from build123d import *

# Parameters (mm, degrees)
F1_DEPTH = 82.55
F2_T     = -3.175
F5_DEPTH = 3.175
F6_DEPTH = 3.175


with BuildPart() as f1:
    # F0 (on Top) → F1 (new body)
    with BuildSketch(Plane.XY):
        Polygon((-132.221535, 93.801795), (-132.221535, 90.626795), (-132.221535, -188.773205), (-132.221535, -191.948205), (115.428465, -191.948205), (115.428465, -188.773205), (115.428465, 93.801795), (112.253465, 93.801795), align=None)
    extrude(amount=F1_DEPTH)

    # F2
    f2_openings = [f1.faces().sort_by_distance(p)[0] for p in [
        (-8.396535, -49.073205, 82.55),
    ]]
    offset(amount=F2_T, openings=f2_openings)

    # F3 (on face) → F5 (join)
    with BuildSketch(Plane.YZ.offset(115.428465)):
        with BuildLine():
            ThreePointArc((52.526795, 53.975), (43.546539, 32.294744), (65.226795, 41.275))
            ThreePointArc((65.226795, 41.275), (61.507051, 50.255256), (52.526795, 53.975))
        make_face()
    extrude(amount=F5_DEPTH)

    # F4 (on face) → F6 (join)
    with BuildSketch(Plane(origin=(-132.221535, 0, 0), x_dir=(0, -1, 0), z_dir=(-1, 0, 0))):
        with BuildLine():
            ThreePointArc((-52.526795, 53.975), (-61.507051, 50.255256), (-65.226795, 41.275))
            ThreePointArc((-65.226795, 41.275), (-52.526795, 28.575), (-39.826795, 41.275))
            ThreePointArc((-39.826795, 41.275), (-43.546539, 50.255256), (-52.526795, 53.975))
        make_face()
    extrude(amount=F6_DEPTH)


solid = f1.part
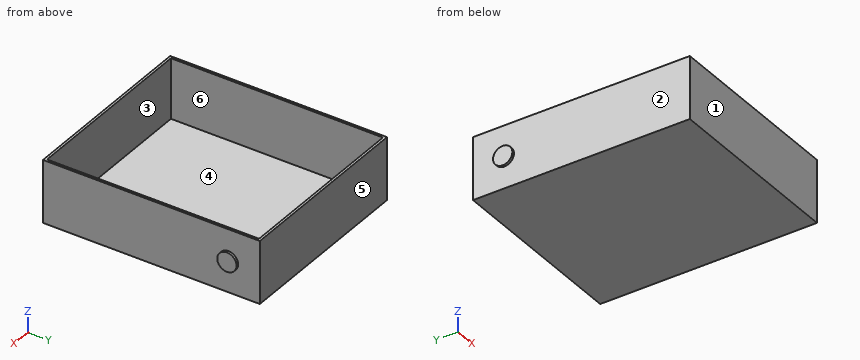
Geometry check sheet. Reference: the model listing, model coordinates, mm. Face numbers are marked on the shaded views. A direction names the side the tool comes from. Give positions to 0.01 mm unless a question says otherwise; leave off trailing zeros. Order: outer loops, then holes, each group sorted by start corner. A loop starts at its lowest first (then second) coordinate and runs counter-clockwise, first axis right, second up.
1) Draft check along X on the marked faces 1, 2, 3 and 4. Enter one of: released by +X, released by -X, zero draft, split by the parting line, or undercut.
Results are:
face 1: zero draft
face 2: released by -X
face 3: undercut
face 4: undercut
2) Cross-section at A-A (z = 72). Record the boundary of the cut face in (x, y).
Results are:
outline: (-132.22, -191.95) - (115.43, -191.95) - (115.43, 93.8) - (-132.22, 93.8) - close; hole (-129.05, -188.77) - (112.25, -188.77) - (112.25, 90.63) - (-129.05, 90.63) - close
3) Material ranges on probe 1 along Y at (x, z) = (-115, 56.5); probe 2 along X at (y, z) = (52.5, 51); probe 3 along X at (y, z) = (-117.5, 34), recorded low to high.
Results are:
probe 1: y = -191.95 to -188.77, 90.63 to 93.8
probe 2: x = -135.4 to -129.05, 112.25 to 118.6
probe 3: x = -132.22 to -129.05, 112.25 to 115.43
4) Gauge pin test, flat ends, axial feed: pin 1 (4 mm diameter, centred on y = -32.5, z = 66, fed in from +X); pin 2 (2 mm diameter, centred on y = 18.5, z = 21.5, fed in from -X); pin 3 (2 mm diameter, centred on x = -18, y = -119, fed in from +Z) (3 decimals). Record the tip position at first contact, or that the pin passes through.
Results are:
pin 1: stops at x = 115.43
pin 2: stops at x = -132.22
pin 3: stops at z = 3.175
5) Cross-section at B-B (y = -130). Record the boundary of the cut face in (x, z) (3 decimals), then the cut area to 3 significant figures.
Results are:
outline: (-132.222, 0) - (115.428, 0) - (115.428, 82.55) - (112.253, 82.55) - (112.253, 3.175) - (-129.047, 3.175) - (-129.047, 82.55) - (-132.222, 82.55) - close
area: 1,290 mm2
6) Cross-section at C-C (x = -44). Record the boundary of the cut face in (y, z) (3 decimals).
Results are:
outline: (-191.948, 0) - (93.802, 0) - (93.802, 82.55) - (90.627, 82.55) - (90.627, 3.175) - (-188.773, 3.175) - (-188.773, 82.55) - (-191.948, 82.55) - close
7) Tool access check on the marked faces 5 and 6. Record the directions out of +Z, -Z, +X, -X, +Y, -Y that give a thin tool (end or side, any length) a straight path to the whole face; none if there is none.
Results are:
face 5: +Z, -Z, +X, -X, +Y
face 6: +Z
8) Cross-section at D-D (z = 36.5). Record the boundary of the cut face in (x, y), then the cut area to 3 significant figures.
Results are:
outline: (-135.4, 40.76) - (-132.22, 40.76) - (-132.22, -191.95) - (115.43, -191.95) - (115.43, 40.76) - (118.6, 40.76) - (118.6, 64.29) - (115.43, 64.29) - (115.43, 93.8) - (-132.22, 93.8) - (-132.22, 64.29) - (-135.4, 64.29) - close; hole (-129.05, -188.77) - (112.25, -188.77) - (112.25, 90.63) - (-129.05, 90.63) - close
area: 3,500 mm2
